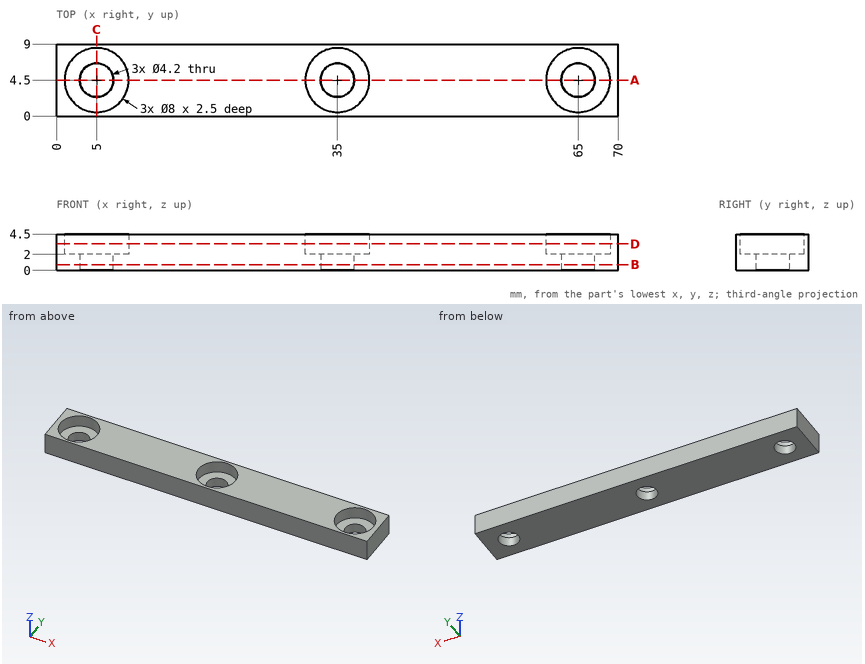
Source: three-view drawing plus pictorial views. Frame: mm from the lowest corner of the part. Coordinates: 2 decimals unless noted, no trailing zeros. Order: outer loops, then holes, each group sorted by start corner. A loop starts at its lowest first (then second) coordinate and runs counter-clockwise, first axis right, second up.
Item 1: Cut plane B-B (z = 0.7). Return loops of the section in (x, y), plus the area to 3 significant figures.
Output values:
outline: (0, 0) - (70, 0) - (70, 9) - (0, 9) - close; hole circle Ø4.2 at (5, 4.5); hole circle Ø4.2 at (35, 4.5); hole circle Ø4.2 at (65, 4.5)
area: 588 mm2
Item 2: Cut plane C-C (x = 5). Return loops of the section in (y, z), plus the area to 3 significant figures.
Output values:
outline: (0, 0) - (2.4, 0) - (2.4, 2) - (0.5, 2) - (0.5, 4.5) - (0, 4.5) - close; (6.6, 0) - (9, 0) - (9, 4.5) - (8.5, 4.5) - (8.5, 2) - (6.6, 2) - close
area: 12.1 mm2
Item 3: Material intervals for line 1 (X direction, y = 4.5, z = 1.3); line 2 (X direction, y = 4, z = 3.4); line 3 (Y direction, x = 65, z = 3.9), sorted ascending.
Output values:
line 1: x = 0 to 2.9, 7.1 to 32.9, 37.1 to 62.9, 67.1 to 70
line 2: x = 0 to 1.03, 8.97 to 31.03, 38.97 to 61.03, 68.97 to 70
line 3: y = 0 to 0.5, 8.5 to 9
Item 4: Cut plane D-D (z = 3.3). Return loops of the section in (x, y).
Output values:
outline: (0, 0) - (70, 0) - (70, 9) - (0, 9) - close; hole circle Ø8 at (5, 4.5); hole circle Ø8 at (35, 4.5); hole circle Ø8 at (65, 4.5)
Item 5: First-contact query: P1, Ø4, axis at x = 64, y = 4.5, coming from the +Z side; P2, Ø2.5, axis at x = 65, y = 4.5, coming from the -Z side. Flat tips, straight axial feed; report the tip coordinate or a pass-through.
Output values:
P1: stops at z = 2
P2: passes through
Item 6: Cut plane A-A (y = 4.5). Return loops of the section in (x, z), plus the area to 3 significant figures.
Output values:
outline: (0, 0) - (2.9, 0) - (2.9, 2) - (1, 2) - (1, 4.5) - (0, 4.5) - close; (7.1, 0) - (32.9, 0) - (32.9, 2) - (31, 2) - (31, 4.5) - (9, 4.5) - (9, 2) - (7.1, 2) - close; (37.1, 0) - (62.9, 0) - (62.9, 2) - (61, 2) - (61, 4.5) - (39, 4.5) - (39, 2) - (37.1, 2) - close; (67.1, 0) - (70, 0) - (70, 4.5) - (69, 4.5) - (69, 2) - (67.1, 2) - close
area: 230 mm2
